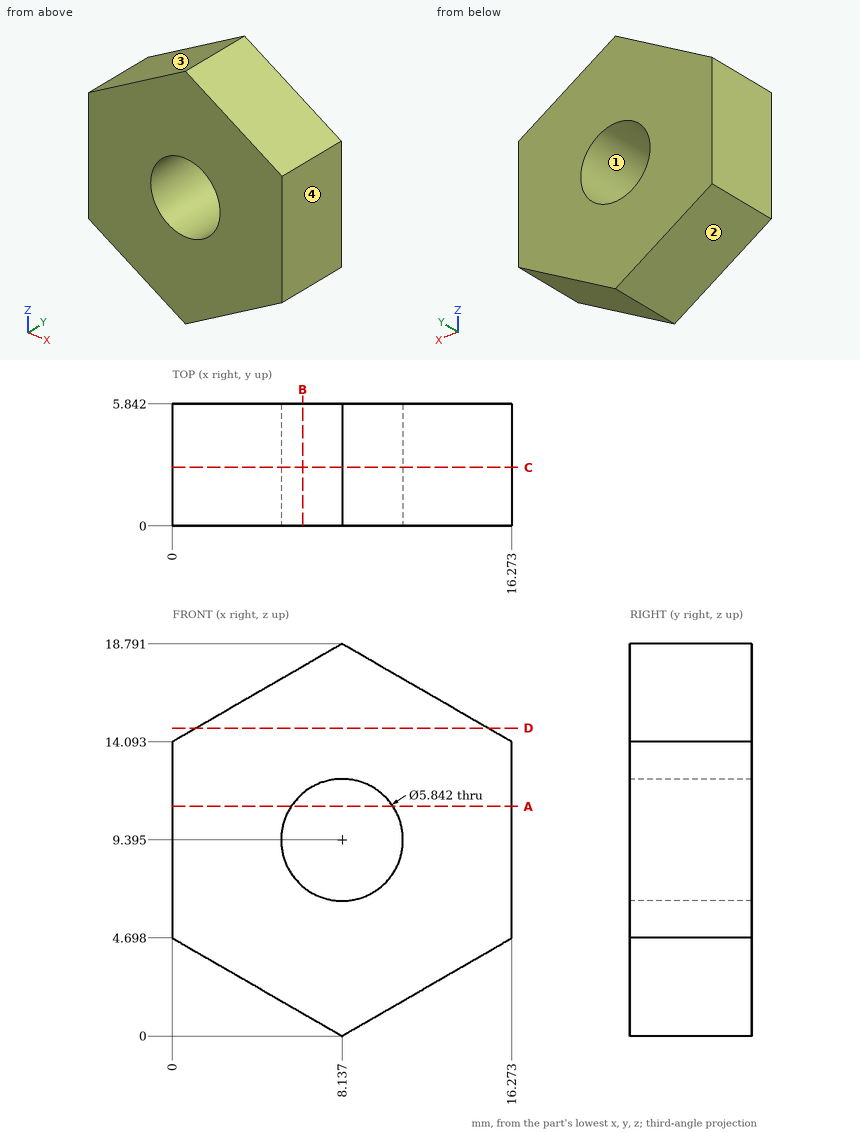
Part print with two shaded views. Sizes in mm from the minimum x, y, z corner. Coordinates: 2 decimals unless noted, no trailing zeros. Loops run counter-clockwise (first coordinate to the right, second up) from the corner with the lowest first, then second, coordinate; pieces in that order, holes last. Notation, with made-up numbers: (-31.5, 77) - (1.5, 77) arc R28 ccw to (1.5, 95) - close; hole circle Ø9 at (69.25, -24). An arc over 180 degrees is marked (long way). Write each question's results on one line, items separated by ' | '. Start each with the question number.
Q1. Slice it at D-D on z = 14.75. Give the cut face in (x, y) (1 decimal).
Q2. Slice it at A-A on z = 11. Give the cut face in (x, y).
Q3. Slice it at B-B on x = 6.25. Give the cut face in (y, z) (1 decimal).
Q4. Two-plate mould, pull along Z, no slides. Class the marked faces 1, 2, 3 and 4: +Z half, -Z half, draft (parallel to the pull), parting line (faces both ways), or undercut.
Q5. Drop flat-ended pins along their axis: pin 1 Ø2 at (x, y) = (2, 3.5) entering from +Z (1 decimal); pin 2 Ø1.5 at (x, y) = (4, 1) entering from -Z (1 decimal); pin 3 Ø2 at (x, y) = (3, 5) entering from +Z. Give the stop position or say it passes through.
Q6. Slice it at C-C on y = 2.8. Give the cut face in (x, z) (1 decimal).
Q7. Probe line 1 along Z through (x, y) = (7, 2.7) (1 decimal); line 2 along X through (y, z) = (3.85, 11) (1 decimal); line 3 along Z through (x, y) = (7.5, 1.2) (1 decimal). List the from-to ranges inside material, lowest first.
Answer:
1) outline: (1.1, 0) - (15.1, 0) - (15.1, 5.8) - (1.1, 5.8) - close
2) outline: (0, 0) - (5.7, 0) - (5.7, 5.84) - (0, 5.84) - close; (10.58, 0) - (16.27, 0) - (16.27, 5.84) - (10.58, 5.84) - close
3) outline: (0, 1.1) - (5.8, 1.1) - (5.8, 7.2) - (0, 7.2) - close; (0, 11.6) - (5.8, 11.6) - (5.8, 17.7) - (0, 17.7) - close
4) face 1: undercut | face 2: -Z half | face 3: +Z half | face 4: draft
5) pin 1: stops at z = 15.8 | pin 2: stops at z = 2 | pin 3: stops at z = 16.4
6) outline: (0, 4.7) - (8.1, 0) - (16.3, 4.7) - (16.3, 14.1) - (8.1, 18.8) - (0, 14.1) - close; hole circle Ø5.8 at (8.1, 9.4)
7) line 1: z = 0.7 to 6.7, 12.1 to 18.1 | line 2: x = 0 to 5.7, 10.6 to 16.3 | line 3: z = 0.4 to 6.5, 12.2 to 18.4
